The listing builds one solid part. Answer for the finished solid, in the listing's coordinates (mm). Coordinates: 2 decimals unless noted, no trailing zeros. Write each loop counter-clockwise with the first axis right and the second up, starting at its lowest first coordinate (ties: lowest second). Pieces come first, ordered by that corner, then holes. Notation, with made-up numbers: M -23,-3.75 L 3,-3.75 A24 ccw 3,13.25 Z; hole C 30.5,43.5 d10. An arc over 180 degrees is marked long. Answer as CSV lines item,"result".
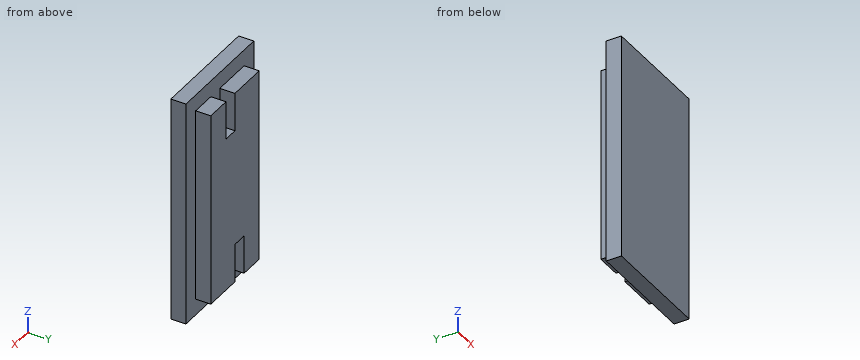
```python
from build123d import *

# Parameters (mm, degrees)
SKETCH1_W           = 15
SKETCH1_H           = 30
BOSS_EXTRUDE1_DEPTH = 2
SKETCH2_W           = 10.7
SKETCH2_H           = 25.7
BOSS_EXTRUDE2_DEPTH = 2
SKETCH3_W           = 2
SKETCH3_H           = 5.1
CUT_EXTRUDE1_DEPTH  = 2


with BuildPart() as part:
    # Sketch1 → Boss-Extrude1 (new body)
    with BuildSketch(Plane(origin=(0, 0, 0), x_dir=(1, 0, 0), z_dir=(0, 1, 0))):
        with Locations((7.5, 15)):
            Rectangle(SKETCH1_W, SKETCH1_H)
    extrude(amount=BOSS_EXTRUDE1_DEPTH)

    # Sketch2 → Boss-Extrude2 (add)
    with BuildSketch(Plane(origin=(0, 2, 0), x_dir=(1, 0, 0), z_dir=(0, 1, 0))):
        with Locations((7.5, 15)):
            Rectangle(SKETCH2_W, SKETCH2_H)
    extrude(amount=BOSS_EXTRUDE2_DEPTH)

    # Sketch3 → Cut-Extrude1 (cut)
    with BuildSketch(Plane(origin=(0, 4, 0), x_dir=(1, 0, 0), z_dir=(0, 1, 0))):
        with Locations((6.5, 25.3)):
            Rectangle(SKETCH3_W, SKETCH3_H)
        with Locations((8.5, 4.7)):
            Rectangle(SKETCH3_W, SKETCH3_H)
    extrude(amount=-CUT_EXTRUDE1_DEPTH, mode=Mode.SUBTRACT)


solid = part.part
```
Q1. Straight lines are drawn through the part: line 1 (X direction, y = 3.4, z = -25.75); line 2 (Z direction, x = 10, y = 3.4); line 3 (X direction, y = 2.2, z = -21.75). For each, find the intervals that lie inside material, in ascending order.
Output:
line 1,"2.15 to 5.5, 7.5 to 12.85"
line 2,"-27.85 to -2.15"
line 3,"2.15 to 12.85"
Q2. Find section A-A (z = -2.5). Give the vertices of the cut face in (x, y), and give its area (3 significant figures).
Output:
outline,"M 0,0 L 15,0 L 15,2 L 12.85,2 L 12.85,4 L 9.5,4 L 9.5,2 L 7.5,2 L 7.5,4 L 2.15,4 L 2.15,2 L 0,2 Z"
area,"47.4 mm2"
Q3. Flat-ended cylindrical pins translate along their axes: pin 1 Ø0.6 at (x, y) = (11, 3.5) entering from +Z; pin 2 Ø1.5 at (y, z) = (3.5, -20) entering from -X; pin 3 Ø2 at (y, z) = (3.5, -24) entering from +X. Find the tip coordinate at first contact, or state that the pin passes through.
Output:
pin 1,"z = -2.15"
pin 2,"x = 2.15"
pin 3,"x = 12.85"
Q4. Find section C-C (y = 2.6). Give the vertices of the cut face in (x, z), and give its area (3 significant figures).
Output:
outline,"M 2.15,-27.85 L 5.5,-27.85 L 5.5,-22.75 L 7.5,-22.75 L 7.5,-27.85 L 12.85,-27.85 L 12.85,-2.15 L 9.5,-2.15 L 9.5,-7.25 L 7.5,-7.25 L 7.5,-2.15 L 2.15,-2.15 Z"
area,"255 mm2"
Q5. Find section B-B (x = 5). Give the vertices of the cut face in (y, z).
Output:
outline,"M 0,-30 L 2,-30 L 2,-27.85 L 4,-27.85 L 4,-2.15 L 2,-2.15 L 2,0 L 0,0 Z"
Q6. Find section D-D (z = -10). Give the vertices of the cut face in (x, y), and give its area (3 significant figures).
Output:
outline,"M 0,0 L 15,0 L 15,2 L 12.85,2 L 12.85,4 L 2.15,4 L 2.15,2 L 0,2 Z"
area,"51.4 mm2"
